Autodesk Inventor part; units mm, degrees
ref_plane "YZ Plane" through (0, 0, 0) normal (1, 0, 0) x (0, 1, 0)
ref_plane "XZ Plane" through (0, 0, 0) normal (0, 1, 0) x (-1, 0, 0)
ref_plane "XY Plane" through (0, 0, 0) normal (0, 0, 1) x (1, 0, 0)
sketch "Skizze1" plane through (0, 0, 0) normal (0, 0, 1) x (1, 0, 0)
  line L0 (-30, -80) -> (30, -80)
  line L1 (30, -80) -> (30, 80)
  line L2 (30, 80) -> (-30, 80)
  line L3 (-30, 80) -> (-30, -80)
  line L4 (-30, -80) -> (30, 80) construction
  line L5 (30, -80) -> (-30, 80) construction
  point P0 (0, 0)
  dimension "d0" = 60
  dimension "d1" = 160
extrude "Extrusion1" add sketch "Skizze1" along normal blind 100
sketch "Skizze2" plane through (30, -80, 0) normal (1, 0, 0) x (0, 0, -1)
  line L0 (-100, 160) -> (-100, 0)
  line L1 (0, 0) -> (-100, 0)
  line L2 (-100, 160) -> (-100, 0)
  line L3 (-100, 0) -> (-130, 0)
  spline S0 degree 4 poles (-130, 0) (-130, 41.0456) (-115, 80) (-100, 118.9544) (-100, 160) knots 0 0 0 0 0 1 1 1 1 1
  point P0 (0, 80)
  point P1 (-115, 80)
  point P2 (-100, 80)
  point P3 (-115, 0)
  dimension "d4" = 30
extrude "Extrusion2" add sketch "Skizze2" against normal up to surface (60 mm away)
sketch "Skizze5" plane through (30, -80, 0) normal (1, 0, 0) x (0, 0, -1)
  line L0 (0, 0) -> (-70, 0)
  line L1 (-70, 0) -> (-70, 13)
  line L2 (-70, 13) -> (0, 13)
  line L3 (0, 13) -> (0, 0)
  point P0 (0, 80)
  dimension "d15" = 70
  dimension "d16" = 13
extrude "Extrusion5" cut sketch "Skizze5" against normal through all
sketch "Skizze6" plane through (30, 80, 100) normal (1, 0, 0) x (0, 0, -1)
  line L0 (30, -160) -> (-30, -160)
  line L1 (10, -160) -> (10, -190)
  line L2 (10, -190) -> (-30, -190)
  line L3 (-30, -190) -> (-30, -160)
  line L4 (30, -160) -> (30, -147)
  line L5 (100, 0) -> (0, 0)
  line L6 (0, 0) -> (30, 0)
  line L7 (30, 0) -> (30, 12)
  line L8 (30, 12) -> (0, 12)
  line L9 (0, 12) -> (0, 0)
  point P0 (100, -80)
  point P1 (30, 0)
  dimension "d19" = 20
  dimension "d20" = 40
  dimension "d21" = 30
  dimension "d24" = 30
  dimension "d25" = 12
extrude "Extrusion6" add sketch "Skizze6" against normal up to surface (60 mm away)
fillet "Rundung1" radius 10 2 edges at (0, -67, 0) (0, 80, 0)
equation "\"G_L\" = 0"
equation "\"G_H\" = 0"
equation "\"G_B\" = 0"
properties part number "canopy" material "GEDA Polyamid schwarz"
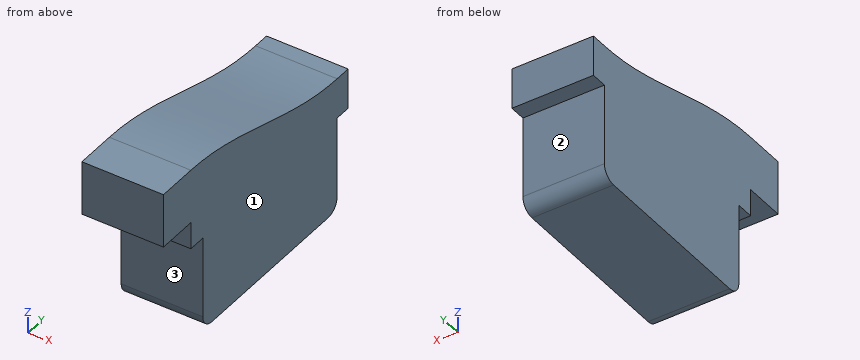
For this review, take the finished solid that the model builds, in its own axes (mm). Face numbers are marked on the shaded views. A direction names the side the tool comes from. Coordinates: 2 decimals unless noted, no trailing zeros. Order: outer loops, then holes, each group sorted by start corner. A loop starts at its lowest first (then second) coordinate and runs counter-clockwise, first axis right, second up. Notation, with made-up numbers: (88.5, 6) - (141.5, 6) arc R27 cw to (141.5, 32) - close; hole circle Ø3 at (-15.5, 28.5). An arc over 180 degrees is marked (long way). Answer as a JSON object with one key per item and string values. Group by question number.
1. For the marked faces 1, 2 and 3, list the 3-axis set-ups (+Z, -Z, +X, -X, +Y, -Y) from which the entire face can be reached by the end or side of a thin tool; tool diameter is ignored.
2. Clearance check with flat-ended pins moving along their axes: P1, Ø14.5, axis at x = 6.5, y = -71.5, coming from the -Z side; P2, Ø6, axis at x = 15, z = 78, coming from the -Y side; P3, Ø10, axis at x = -14, z = 55, coming from the +Y side. State where each tip first meets the part, or that it passes through.
3. We need section A-A on z = 81. State the section outline as (x, y) points.
4. For probe 1 along Y at (x, z) = (-19.5, 48); probe 2 along Y at (x, z) = (-24, 80.5); probe 3 along Z at (x, y) = (-15, -90.5), list the stretches that pass through material, from the lowest coordinate up.
5. We need section B-B on z = 43.5. State the section outline as (x, y) points, then the cut area to 3 significant figures.
Final values:
{
 "1": {"face 1": "+Z, -Z, +X, +Y, -Y", "face 2": "-Z, +X, -X, +Y", "face 3": "-Z, +X, -X, -Y"},
 "2": {"P1": "z = 3.11", "P2": "y = -80", "P3": "y = 80"},
 "3": {"outline": "(-30, -80) - (30, -80) - (30, 92) - (-30, 92) - close"},
 "4": {"probe 1": "-67 to 80", "probe 2": "-80 to 92", "probe 3": "90 to 130"},
 "5": {"outline": "(-30, -67) - (30, -67) - (30, 80) - (-30, 80) - close", "area": "8,820 mm²"}
}
